```python
from build123d import *

# Parameters (mm, degrees)
SKETCH1_R           = 101.6
SKETCH1_R_2         = 57.15
BOSS_EXTRUDE1_DEPTH = 6.35


with BuildPart() as part:
    # Sketch1 → Boss-Extrude1 (new body)
    with BuildSketch(Plane(origin=(0, 0, 0), x_dir=(1, 0, 0), z_dir=(0, 1, 0))):
        Polygon((0, 0), (0, -50.8), (-508, -50.8), (-508, 0), (-558.8, 0), (-558.8, 406.4), (-508, 406.4), (-508, 457.2), (0, 457.2), (0, 406.4), (50.8, 406.4), (50.8, 0), align=None)
        with Locations((-419.1, 152.4)):
            Circle(SKETCH1_R, mode=Mode.SUBTRACT)
        with Locations((-88.9, 152.4)):
            Circle(SKETCH1_R, mode=Mode.SUBTRACT)
        with Locations((-254, 345.42328875)):
            Circle(SKETCH1_R_2, mode=Mode.SUBTRACT)
    extrude(amount=BOSS_EXTRUDE1_DEPTH)


solid = part.part
```
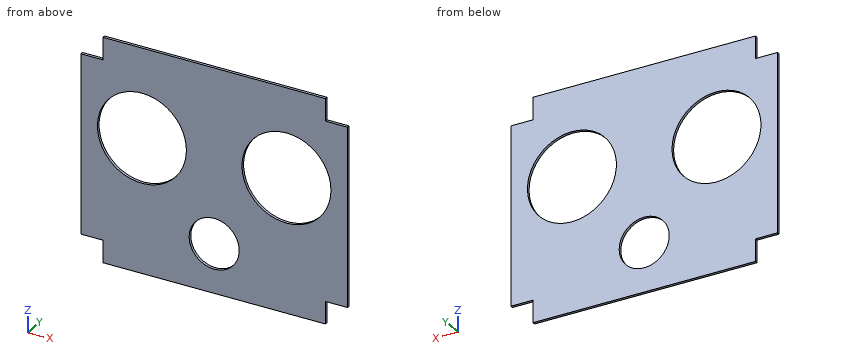
Check sheet for the modelled part. Datum: model origin and axes. Units: mm. Give positions to 0.01 mm unless a question says otherwise; leave off trailing zeros. Order: outer loops, then holes, each group sorted by start corner. A loop starts at its lowest first (then second) coordinate and runs counter-clockwise, first axis right, second up. Notation, with made-up numbers: M 25.5,62.5 L 56.5,62.5 A7 cw 56.5,66.5 Z; hole C 88,-3 d3. An arc over 180 degrees is marked long. Answer in a Markdown table with one row per item. Add a question column.
Q1. Sectioned sample at A-A, the plane z = -152.4. Record the boundary of the cut face in (x, y).
Q2. Sectioned sample at D-D, the plane y = 4.25. Record the boundary of the cut face in (x, z), and give its area (3 significant figures).
Q3. Sectioned sample at B-B, the plane x = -419.1. Record the boundary of the cut face in (y, z).
Q4. Thickness scan on L1, parallel to X at y = 4.5, z = -157.5; L2, parallel to X at y = 4.5, z = -152.4; L3, parallel to Z at x = -254, y = 3. Record the ranges inside material, lowest first.
Q5. Sectioned sample at C-C, the plane z = -389.5. Record the boundary of the cut face in (x, y).
Q6. Gauge pin test, flat ends, axial feed: pin 1 Ø1.9 at (y, z) = (3, 27.5) entering from -X; pin 2 Ø3 at (x, y) = (16.5, 4) entering from +Z; pin 3 Ø1.9 at (y, z) = (3.5, -436.5) entering from +X. Record the tip position at first contact, or that the pin passes through.
Verdict:
| question | item | result |
|---|---|---|
| 1 | outline | M -558.8,0 L -520.7,0 L -520.7,6.35 L -558.8,6.35 Z; M -317.5,0 L -190.5,0 L -190.5,6.35 L -317.5,6.35 Z; M 12.7,0 L 50.8,0 L 50.8,6.35 L 12.7,6.35 Z |
| 2 | outline | M -558.8,-406.4 L -508,-406.4 L -508,-457.2 L 0,-457.2 L 0,-406.4 L 50.8,-406.4 L 50.8,0 L 0,0 L 0,50.8 L -508,50.8 L -508,0 L -558.8,0 Z; hole C -419.1,-152.4 d203.2; hole C -254,-345.42 d114.3; hole C -88.9,-152.4 d203.2 |
| 2 | area | 224,000 mm² |
| 3 | outline | M 0,-457.2 L 6.35,-457.2 L 6.35,-254 L 0,-254 Z; M 0,-50.8 L 6.35,-50.8 L 6.35,50.8 L 0,50.8 Z |
| 4 | L1 | -558.8 to -520.57, -317.63 to -190.37, 12.57 to 50.8 |
| 4 | L2 | -558.8 to -520.7, -317.5 to -190.5, 12.7 to 50.8 |
| 4 | L3 | -457.2 to -402.57, -288.27 to 50.8 |
| 5 | outline | M -558.8,0 L -290.38,0 L -290.38,6.35 L -558.8,6.35 Z; M -217.62,0 L 50.8,0 L 50.8,6.35 L -217.62,6.35 Z |
| 6 | pin 1 | x = -508 |
| 6 | pin 2 | z = 0 |
| 6 | pin 3 | x = 0 |
